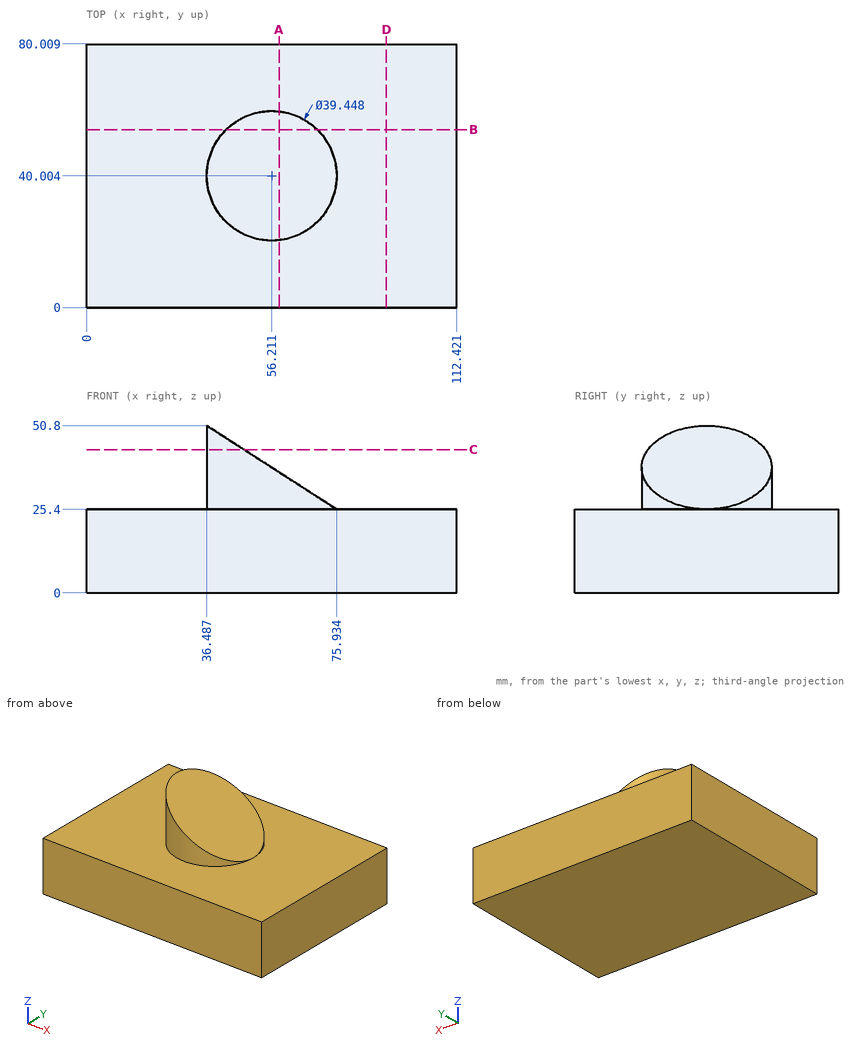
Here's the drawing with two shaded views (mm, measured from the low corner). I have some questions. Give positions to 0.01 mm unless a question says otherwise; leave off trailing zeros. Write each loop counter-clockwise with the first axis right and the second up, starting at its lowest first coordinate (ties: lowest second). Pieces come first, ordered by that corner, then holes. Notation, with made-up numbers: (-32.5, -26.5) -> (-6.5, -26.5) arc R17 ccw to (-6.5, -20.5) -> close; hole circle Ø5 at (30.5, 42.25). An arc over 180 degrees is marked (long way). Use one line per item in the form item = value. Start each with the question number.
1. If I drill on L1, parallel to Y at x = 55.5, z = 36 (1 decimal); L2, parallel to Z at x = 39.5, y = 18.5; L3, parallel to Z at x = 64.5, y = 26.5, over which ranges is the centre line in solid material (lowest first)?
2. Imagine slicing it at B-B on y = 54. List the corners of the cut face in (x, z) for me, plus the area to 3 significant figures.
3. Imagine slicing it at D-D on x = 91. List the corners of the cut face in (y, z) for me, plus the area to 3 significant figures.
4. Will these pins go through, and if not, where does the flat tip stop? pin 1 Ø1.5 at (x, y) = (92, 38.5) entering from +Z; pin 2 Ø5 at (y, z) = (50, 31.5) entering from +X (1 decimal); pin 3 Ø5 at (x, z) = (45.5, 28.5) entering from +Y.
5. Imagine slicing it at C-C on z = 43.5. List the corners of the cut face in (x, y) for me (1 decimal).
6. Imagine slicing it at A-A on x = 58.5. List the corners of the cut face in (y, z) for me (1 decimal), plus the area to 3 significant figures.
Entries:
q1.L1 = 20.3 to 59.7
q1.L2 = 0 to 25.4
q1.L3 = 0 to 32.76
q2.outline = (0, 0) -> (112.42, 0) -> (112.42, 25.4) -> (70.11, 25.4) -> (70.11, 29.15) -> (42.31, 47.05) -> (42.31, 25.4) -> (0, 25.4) -> close
q2.area = 3,210 mm²
q3.outline = (0, 0) -> (80.01, 0) -> (80.01, 25.4) -> (0, 25.4) -> close
q3.area = 2,030 mm²
q4.pin_1 = 25.4
q4.pin_2 = 70.3
q4.pin_3 = 57.94
q5.outline = (47.8, 22.2) -> (47.8, 57.9) arc R19.7 ccw to start
q6.outline = (0, 0) -> (80, 0) -> (80, 25.4) -> (59.6, 25.4) -> (59.6, 36.6) -> (20.4, 36.6) -> (20.4, 25.4) -> (0, 25.4) -> close
q6.area = 2,470 mm²
